Design review of the part built by this model. Coordinates are the model's own, in mm. A direction names the side the tool comes from. Coordinates: 2 decimals unless noted, no trailing zeros. Write each loop counter-clockwise with the first axis right and the second up, starting at its lowest first coordinate (ties: lowest second). Pieces come first, ordered by that corner, then holes. Notation, with made-up numbers: M 1.25,4 L 23.25,4 A23 ccw 23.25,18 Z; hole C -16,42.5 d11. An arc over 180 degrees is marked long. Write item = value, one per line.
```python
from build123d import *

# Parameters (mm, degrees)
SKETCH1_W           = 47.5234
SKETCH1_H           = 20.32
BOSS_EXTRUDE1_DEPTH = 1.524
SKETCH2_W           = 20.254011441
SKETCH2_H           = 40.259
BOSS_EXTRUDE2_DEPTH = 1.524
SKETCH3_W           = 20.355556003
SKETCH3_H           = 40.259
BOSS_EXTRUDE3_DEPTH = 1.524
SKETCH5_R           = 3.81
CUT_EXTRUDE1_DEPTH  = 66.421937049


with BuildPart() as part:
    # Sketch1 → Boss-Extrude1 (new body)
    with BuildSketch(Plane(origin=(0, 0, 0), x_dir=(1, 0, 0), z_dir=(0, 1, 0))):
        Rectangle(SKETCH1_W, SKETCH1_H)
    extrude(amount=BOSS_EXTRUDE1_DEPTH)

    # Sketch2 → Boss-Extrude2 (add)
    with BuildSketch(Plane(origin=(-23.749, 0, 0), x_dir=(0, 0, -1), z_dir=(1, 0, 0))):
        with Locations((0.087917198, 20.1295)):
            Rectangle(SKETCH2_W, SKETCH2_H)
    extrude(amount=-BOSS_EXTRUDE2_DEPTH)

    # Sketch3 → Boss-Extrude3 (add)
    with BuildSketch(Plane(origin=(23.749, 0, 0), x_dir=(0, 0, -1), z_dir=(1, 0, 0))):
        with Locations((0.014847815, 20.1295)):
            Rectangle(SKETCH3_W, SKETCH3_H)
    extrude(amount=BOSS_EXTRUDE3_DEPTH)

    # Sketch5 → Cut-Extrude1 (cut, through all)
    with BuildSketch(Plane.ZY.offset(25.273)):
        with Locations((-0.107211081, 26.738775407)):
            Circle(SKETCH5_R)
    extrude(amount=-CUT_EXTRUDE1_DEPTH, mode=Mode.SUBTRACT)


solid = part.part
```
Q1. Consider section A-A, the plane y = 17.5. State the section outline as (x, z) points, and give its area (3 significant figures).
Check result:
outline = M -25.27,-10.21 L -23.75,-10.21 L -23.75,10.04 L -25.27,10.04 Z; M 23.75,-10.19 L 25.27,-10.19 L 25.27,10.16 L 23.75,10.16 Z
area = 61.9 mm²
Q2. Wall thickness on line 1 (X direction, y = 38, z = -2.25); line 2 (Y direction, x = 23.5, z = -8): over which ranges is each line inside the solid? List them lowest first.
Check result:
line_1 = -25.27 to -23.75, 23.75 to 25.27
line_2 = 0 to 1.52
Q3. Consider section D-D, the plane z = -7. State the section outline as (x, y) points, and give its area (3 significant figures).
Check result:
outline = M -25.27,0 L 25.27,0 L 25.27,40.26 L 23.75,40.26 L 23.75,1.52 L -23.75,1.52 L -23.75,40.26 L -25.27,40.26 Z
area = 195 mm²
Q4. Machinability: for faces 5 (the flat face through (23.749, 20, 0)), 6 (the flat face through (-25, 40.259, 0)), which of the approach directions +Z, -Z, +X, -X, +Y, -Y give a long, thin tool a straight path to every point of the face, cutting with its end or side? Answer none if there is none.
Check result:
face_5 = +Z, -Z, +Y
face_6 = +Z, -Z, +X, -X, +Y
Q5. For P1, Ø1.7, axis at x = -4, y = 1, coming from the -Z side; P2, Ø1.7, axis at x = -24.5, y = 14.5, coming from the +Z side; P3, Ø4, axis at x = -20, y = 4, coming from the +Z side; P4, Ø1.7, axis at x = -10, y = 0.5, coming from the +Z side, all flat-tipped, find the tip position at first contact; note any pin that passes through.
Check result:
P1 = -10.16
P2 = 10.04
P3 = through
P4 = 10.16
Q6. Consider section C-C, the plane y = 28.5. State the section outline as (x, z) points, and give its area (3 significant figures).
Check result:
outline = M -25.27,-10.21 L -23.75,-10.21 L -23.75,-3.49 L -25.27,-3.49 Z; M -25.27,3.27 L -23.75,3.27 L -23.75,10.04 L -25.27,10.04 Z; M 23.75,-10.19 L 25.27,-10.19 L 25.27,-3.49 L 23.75,-3.49 Z; M 23.75,3.27 L 25.27,3.27 L 25.27,10.16 L 23.75,10.16 Z
area = 41.3 mm²
Q7. Consider section B-B, the plane z = -1.25. State the section outline as (x, y) points.
Check result:
outline = M -25.27,0 L 25.27,0 L 25.27,23.1 L 23.75,23.1 L 23.75,1.52 L -23.75,1.52 L -23.75,23.1 L -25.27,23.1 Z; M -25.27,30.37 L -23.75,30.37 L -23.75,40.26 L -25.27,40.26 Z; M 23.75,30.37 L 25.27,30.37 L 25.27,40.26 L 23.75,40.26 Z
Q8. The part is to be moulded in two halves that separate along Y. For faces 1 (the cylindrical face through (-24.522, 30.516, -0.603)), 2 (the flat face through (25, 20, 10.163)), 3 (the cylindrical face through (24.5, 30.516, -0.603)), 4 (the flat face through (0, 1.524, 0)), say which applies: +Y half, -Y half, draft (parallel to the pull), parting line (faces both ways), or undercut.
Check result:
face_1 = undercut
face_2 = draft
face_3 = undercut
face_4 = +Y half
